Can you work these out from the model? Positions are in its coordinate system, mm. A direction names the side the tool comes from. Give positions to 0.01 mm unless a question says otherwise; leave off trailing zeros. Loops run counter-clockwise (first coordinate to the right, second up) from the corner with the lowest first, then second, coordinate; pieces in that order, holes last. Notation, with made-up numbers: (-28, 75.5) -> (18, 75.5) arc R21 cw to (18, 96.5) -> close; hole circle Ø3 at (57.25, 24.25). An arc over 180 degrees is marked (long way). Use CSV: the item, a comma, the result in double quotes.
Autodesk Inventor part; units mm, degrees
ref_plane "YZ Plane" through (0, 0, 0) normal (1, 0, 0) x (0, 1, 0)
ref_plane "XZ Plane" through (0, 0, 0) normal (0, 1, 0) x (-1, 0, 0)
ref_plane "XY Plane" through (0, 0, 0) normal (0, 0, 1) x (1, 0, 0)
sketch "スケッチ1" plane through (0, 0, 0) normal (1, 0, 0) x (0, 1, 0)
  circle A0 centre (0, 0) radius 10
  circle A1 centre (0, 0) radius 12.5
  line L0 (3.5, 12.5) -> (-3.5, 12.5)
  line L1 (-3.5, 12.5) -> (-3.5, -12.5)
  line L2 (-3.5, -12.5) -> (3.5, -12.5)
  line L3 (3.5, -12.5) -> (3.5, 12.5)
  line L4 (3.5, 12.5) -> (-3.5, -12.5) construction
  line L5 (-3.5, 12.5) -> (3.5, -12.5) construction
  line L6 (-12.5, 3.5) -> (12.5, 3.5)
  line L7 (12.5, 3.5) -> (12.5, -3.5)
  line L8 (12.5, -3.5) -> (-12.5, -3.5)
  line L9 (-12.5, -3.5) -> (-12.5, 3.5)
  line L10 (-12.5, 3.5) -> (12.5, -3.5) construction
  line L11 (12.5, 3.5) -> (-12.5, -3.5) construction
  point P0 (12, -3.5)
  point P1 (12, 3.5)
  point P2 (3.5, 3.5)
  point P3 (3.5, 12)
  point P4 (-3.5, 12)
  point P5 (-3.5, 3.5)
  point P6 (-12, 3.5)
  point P7 (-12, -3.5)
  point P8 (-3.5, -3.5)
  point P9 (-3.5, -12)
  point P10 (3.5, -12)
  point P11 (3.5, -3.5)
  dimension "d0" = 20
  dimension "d1" = 25
  dimension "d2" = 7
  dimension "d3" = 25
  dimension "d4" = 25
  dimension "d5" = 7
extrude "押し出し1" add sketch "スケッチ1" along normal blind 2 contours A0 L8 L3 L6 | A0 L6 A1 L8 | L3 L6 L1 A0 | A0 L1 A1 L3 | L3 L8 L1 L6 | L3 A1 L1 A0 | A0 L1 L8 L3 | L1 L8 A0 L6 | A0 L8 A1 L6
equation "\"d5\" = d2"
properties part number "RubberSheet_1"
(1) Which directions (+Z, -Z, +X, -X, +Y, -Y) give clear straight access to the entire face, cutting with the end or side of a thin tool? Please do faces 1 (the face through (1, 3.5, -8)), 2 (the face through (1, -8, -3.5)), 3 (the face through (1, -3.5, 8)), 4 (the face through (1, 3.5, 8)).
Answer sheet:
face 1,"-Z, +X, -X, +Y"
face 2,"-Z, +X, -X, -Y"
face 3,"+Z, +X, -X, -Y"
face 4,"+Z, +X, -X, +Y"
(2) Will these pins go through, and if not, where does the flat tip stop? pin 1 Ø1 at (x, y) = (0.5, -7.5) entering from -Z; pin 2 Ø1 at (x, z) = (0.5, 6.5) entering from +Y; pin 3 Ø0.6 at (x, z) = (1.5, 8.5) entering from -Y.
Answer sheet:
pin 1,"stops at z = -3.5"
pin 2,"stops at y = 3.5"
pin 3,"stops at y = -3.5"
(3) If we section it at A-A, the plane x = 0.6: Write out the boundary of the cut face in (y, z).
Answer sheet:
outline,"(-12, -3.5) -> (-3.5, -3.5) -> (-3.5, -12) arc R12.5 ccw to (3.5, -12) -> (3.5, -3.5) -> (12, -3.5) arc R12.5 ccw to (12, 3.5) -> (3.5, 3.5) -> (3.5, 12) arc R12.5 ccw to (-3.5, 12) -> (-3.5, 3.5) -> (-12, 3.5) arc R12.5 ccw to start"
(4) If we section it at B-B, the plane y = -6.5: Write out the boundary of the cut face in (x, z), then the cut area to 3 significant figures.
Answer sheet:
outline,"(0, -3.5) -> (2, -3.5) -> (2, 3.5) -> (0, 3.5) -> close"
area,"14.0 mm2"
(5) If I drill on L1, parallel to Y at x = 0.65, z = -9.75; L2, parallel to Z at x = 1.9, y = -0.25, over which ranges is the centre line in solid material (lowest first)? Write a range as from..to.
Answer sheet:
L1,"y = -3.5..3.5"
L2,"z = -12.5..12.5"
